from build123d import *

# Parameters (mm, degrees)
SKETCH1_R           = 1.778
BOSS_EXTRUDE1_DEPTH = 3.175
SKETCH2_W           = 165.78896247
SKETCH2_H           = 45.115138018
CUT_EXTRUDE1_DEPTH  = 127
SKETCH3_R           = 4.7625
CUT_EXTRUDE2_DEPTH  = 127
SKETCH4_R           = 1.778
CUT_EXTRUDE3_DEPTH  = 127
BOSS_EXTRUDE2_DEPTH = 3.175
FILLET3_R           = 1.27
BOSS_EXTRUDE3_DEPTH = 3.175


with BuildPart() as part:
    # Sketch1 → Boss-Extrude1 (new body)
    with BuildSketch(Plane(origin=(0, 6.35, 0), x_dir=(1, 0, 0), z_dir=(0, 1, 0))):
        with BuildLine():
            Line((187.7568, 6.985), (-187.7568, 6.985))
            ThreePointArc((-187.7568, 6.985), (-194.1068, 0.635), (-187.7568, -5.715))
            Line((-187.7568, -5.715), (187.7568, -5.715))
            ThreePointArc((187.7568, -5.715), (194.1068, 0.635), (187.7568, 6.985))
        make_face()
        with Locations(Location((187.7568, 0.635, 0), (0, 0, 90))):
            Circle(SKETCH1_R, mode=Mode.SUBTRACT)
        with Locations(Location((-187.7568, 0.635, 0), (0, 0, 90))):
            Circle(SKETCH1_R, mode=Mode.SUBTRACT)
    extrude(amount=-BOSS_EXTRUDE1_DEPTH)

    # Sketch2 → Cut-Extrude1 (cut)
    with BuildSketch(Plane(origin=(0, 6.35, 0), x_dir=(1, 0, 0), z_dir=(0, 1, 0))):
        with Locations((-124.419845051, -4.918181187)):
            Rectangle(SKETCH2_W, SKETCH2_H)
    extrude(amount=-CUT_EXTRUDE1_DEPTH, mode=Mode.SUBTRACT)

    # Sketch3 → Cut-Extrude2 (cut)
    with BuildSketch(Plane(origin=(0, 6.35, 0), x_dir=(1, 0, 0), z_dir=(0, 1, 0))):
        with Locations(Location((-35.2044, 0.635, 0), (0, 0, 270))):
            Circle(SKETCH3_R)
    extrude(amount=-CUT_EXTRUDE2_DEPTH, mode=Mode.SUBTRACT)

    # Sketch4 → Cut-Extrude3 (cut)
    with BuildSketch(Plane(origin=(0, 6.35, 0), x_dir=(1, 0, 0), z_dir=(0, 1, 0))):
        with Locations(Location((168.1988, 0.635, 0), (0, 0, 270))):
            Circle(SKETCH4_R)
        with Locations(Location((177.9778, 0.635, 0), (0, 0, 270))):
            Circle(SKETCH4_R)
    extrude(amount=-CUT_EXTRUDE3_DEPTH, mode=Mode.SUBTRACT)

    # Sketch5 → Boss-Extrude2 (add)
    with BuildSketch(Plane(origin=(0, 6.35, 0), x_dir=(1, 0, 0), z_dir=(0, 1, 0))):
        Polygon((-27.555842436, 6.985), (-41.525363816, 6.985), (-41.525363816, -5.715), (-27.555842436, -5.715), (-27.555842436, -7.3025), (-41.525363816, -7.3025), (-43.112863816, -7.3025), (-43.112863816, 8.5725), (-41.525363816, 8.5725), (-27.555842436, 8.5725), align=None)
    extrude(amount=-BOSS_EXTRUDE2_DEPTH)

    # Fillet3
    fillet3_edges = [part.edges().sort_by_distance(p)[0] for p in [
        (-43.112863816, 4.7625, 7.3025),
        (-43.112863816, 4.7625, -8.5725),
    ]]
    fillet(fillet3_edges, radius=FILLET3_R)

    # Sketch6 → Boss-Extrude3 (add)
    with BuildSketch(Plane(origin=(0, 6.35, 0), x_dir=(1, 0, 0), z_dir=(0, 1, 0))):
        Polygon((-27.555842436, 8.5725), (-10.771352163, 6.985), (-27.555842436, 6.985), align=None)
        Polygon((-27.555842436, -7.3025), (-10.771352163, -5.715), (-27.555842436, -5.715), align=None)
    extrude(amount=-BOSS_EXTRUDE3_DEPTH)


solid = part.part
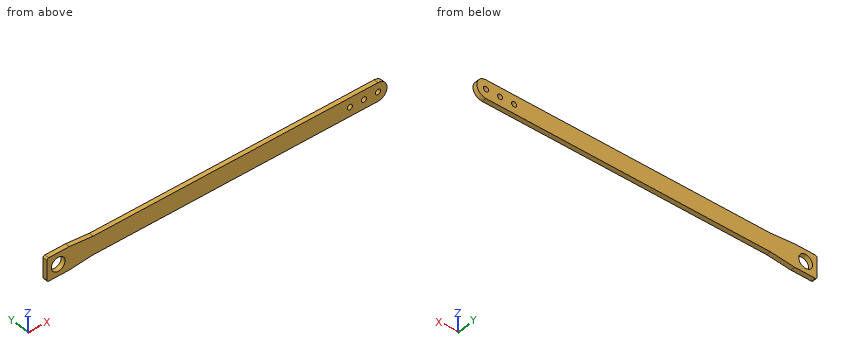
The listing builds one solid part. Answer for the finished solid, in the listing's coordinates (mm). Coordinates: 2 decimals unless noted, no trailing zeros. Order: outer loops, then holes, each group sorted by start corner. A loop starts at its lowest first (then second) coordinate and runs counter-clockwise, first axis right, second up.
Q1. A cutting plane is placed at B-B, the plane x = 62. Write down the section's boundary in (y, z) (3 decimals).
Q2. A cutting plane is placed at A-A, the plane y = 3.85. State how many separate pieces and enclosed holes the cut face has, and give its area (3 significant figures).
Q3. Consider line 1 (X direction, y = 3.5, z = -0.25); line 2 (X direction, y = 5.25, z = -0.5); line 3 (Z direction, x = 32, y = 6.1) (3 decimals). Determine where each line is inside the solid, lowest interval first.
Q4. Given P1, Ø4.5, axis at x = 168.2, z = -0.64, coming from the +Y side; P2, Ø5.5, axis at x = -35.2, z = -0.64, coming from the -Y side; P3, Ø1.5, axis at x = 63.5, y = 4.5, coming from the -Z side (3 decimals), each flat-ended and moving along its own axis, determine where each tip first touches the part or whether it passes through.
Answers follow:
1. outline: (3.175, -6.985) - (6.35, -6.985) - (6.35, 5.715) - (3.175, 5.715) - close
2. separate pieces: 1
2. enclosed holes: 4
2. area: 2,970 mm2
3. line 1: x = -43.11 to -39.95, -30.46 to 166.46, 169.93 to 176.24, 179.71 to 186.02, 189.49 to 194.1
3. line 2: x = -43.11 to -39.96, -30.44 to 166.43, 169.97 to 176.2, 179.75 to 185.98, 189.53 to 194.11
3. line 3: z = -6.985 to 5.715
4. P1: stops at y = 6.35
4. P2: passes through
4. P3: stops at z = -6.985
